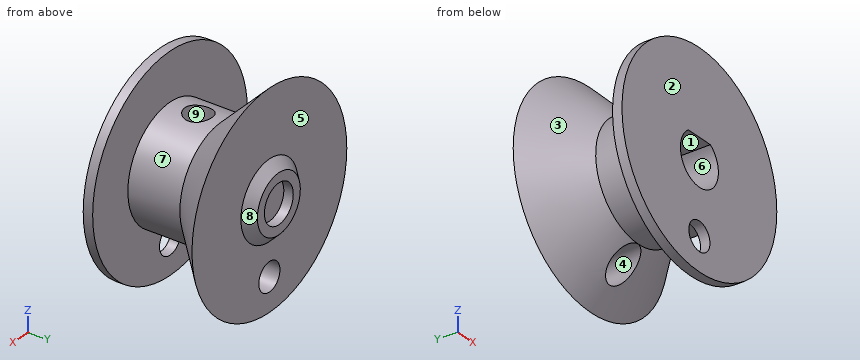
```python
from build123d import *

# Parameters (mm, degrees)
FLATSPOT_EXTRUDE_REACH     = 21.956
WIRE_HOLE_CUT_DEPTH        = 20.345542122
WIRE_HOLE_CUT_DEPTH_BACK   = 20.345542122
SKETCH5_R                  = 1.5
SKETCH6_R                  = 1.425
SET_SCREW_CUT_DEPTH        = 19.1400801
MAGNET_START               = -1
SKETCH8_R                  = 11
SKETCH8_R_2                = 3.05
MAGNET_HOLDER_TRIM_DEPTH   = 1
MAGNET_HOLDER_CHAMFER_SIZE = 1
AXLE_TOLERANCE_CUT_DEPTH   = 8


with BuildPart() as part:
    # Sketch1 → Spool Solid (revolve)
    with BuildSketch(Plane(origin=(0, 0, 0), x_dir=(0, 0, -1), z_dir=(1, 0, 0)), mode=Mode.PRIVATE) as spool_solid_sk:
        Polygon((-11, 6.25), (-11, 5.25), (-6, 0.25), (-6, -5.25), (-11, -5.25), (-11, -6.25), (-2.5, -6.25), (-2.5, 1.75), (0, 4.25), (0, 5.25), (-2.05, 5.25), (-2.05, 6.25), (-2.5, 6.25), align=None)
    revolve(spool_solid_sk.sketch.rotate(Axis((0, 0, 0), (0, 1, 0)), 180), axis=Axis((0, 0, 0), (0, 1, 0)))

    # Flatspot Extrude: up to this cone (the profile starts inside it)
    flatspot_extrude_end = Plane(origin=(0, -6.25, 0), z_dir=(0, -1, 0)).offset(-10.499999) * Cone(1e-06, 43.456, 43.455999, align=(Align.CENTER, Align.CENTER, Align.MIN), mode=Mode.PRIVATE)
    # Sketch2 → Flatspot Extrude (add, up to the surface)
    with BuildSketch(Plane.XZ.offset(6.25), mode=Mode.PRIVATE) as flatspot_extrude_sk1:
        with BuildLine():
            Line((1.5, 2), (-1.5, 2))
            ThreePointArc((-1.5, 2), (0, 2.5), (1.5, 2))
        make_face()
    flatspot_extrude_tool1 = extrude(flatspot_extrude_sk1.sketch, amount=-FLATSPOT_EXTRUDE_REACH, mode=Mode.PRIVATE) & flatspot_extrude_end
    add(flatspot_extrude_tool1.solids().sort_by_distance((0, -6.25, 2.20182))[0])

    # Sketch5 → Wire Hole cut (cut, two sides: drawn at the far end of the back side and taken through both)
    with BuildSketch(Plane(origin=(0, -5.25, 0), x_dir=(1, 0, 0), z_dir=(0, 1, 0)).offset(-WIRE_HOLE_CUT_DEPTH_BACK)):
        with Locations(Location((0, 7.5, 0), (0, 0, 270))):
            Circle(SKETCH5_R)
    extrude(amount=WIRE_HOLE_CUT_DEPTH + WIRE_HOLE_CUT_DEPTH_BACK, mode=Mode.SUBTRACT)

    # Sketch6 → Set Screw Cut (cut, through all)
    with BuildSketch(Plane(origin=(0, 0, 2), x_dir=(-1, 0, 0), z_dir=(0, 0, -1))):
        with Locations((0, -2.25)):
            Circle(SKETCH6_R)
    extrude(amount=-SET_SCREW_CUT_DEPTH, mode=Mode.SUBTRACT)

    # Sketch8 → Magnet Holder Trim (cut)
    with BuildSketch(Plane(origin=(0, 6.25, 0), x_dir=(1, 0, 0), z_dir=(0, 1, 0)).offset(MAGNET_START)):
        with Locations(Location((0, 0, 0), (0, 0, 90))):
            Circle(SKETCH8_R)
        with Locations(Location((0, 0, 0), (0, 0, 270))):
            Circle(SKETCH8_R_2, mode=Mode.SUBTRACT)
    extrude(amount=MAGNET_HOLDER_TRIM_DEPTH, mode=Mode.SUBTRACT)

    # Magnet Holder Chamfer
    magnet_holder_chamfer_edges = [part.edges().sort_by_distance(p)[0] for p in [
        (0, 5.25, -3.05),
    ]]
    chamfer(magnet_holder_chamfer_edges, length=MAGNET_HOLDER_CHAMFER_SIZE - 0.0001)  # a hair under: the kernel refuses the full size

    # Sketch9 → Axle Tolerance Cut (cut)
    with BuildSketch(Plane.XZ.offset(6.25)):
        with BuildLine():
            Line((1.565247584, 2.2), (-1.565247584, 2.2))
            ThreePointArc((-1.565247584, 2.2), (0, -2.7), (1.565247584, 2.2))
        make_face()
    extrude(amount=-AXLE_TOLERANCE_CUT_DEPTH, mode=Mode.SUBTRACT)


solid = part.part
```
CAD build for the part. Positions are in the model's coordinates, mm. Face numbers are marked on the shaded views. A direction names the side the tool comes from. Round coordinates to 2 decimals unless told otherwise and drop trailing zeros. Write each loop counter-clockwise with the first axis right and the second up, starting at its lowest first coordinate (ties: lowest second). Pieces come first, ordered by that corner, then holes. Notation, with made-up numbers: (82, -4) - (139, -4) arc R33 ccw to (139, 34) - close; hole circle Ø10 at (69.25, -1.75). An arc over 180 degrees is marked (long way). Return JSON: item names as keys, results as strings. Group by question number.
Item 1: Probe probe 1 along Y at (x, z) = (0, 10); probe 2 along Z at (x, y) = (0.25, 4.5); probe 3 along Y at (x, z) = (-7.25, -6.75). List the from-to ranges inside material, lowest first.
Item 2: Flat gauge pins, fed straight in: pin 1 Ø4 at (x, z) = (0, -7.5) entering from +Y; pin 2 Ø3.5 at (x, y) = (0, -2.25) entering from -Z; pin 3 Ø5 at (x, y) = (4.5, -5) entering from -Z. Where does each tip first touch, or does it go through?
Item 3: Band-saw the part on B-B on y = -2.25. List the corners of the cut face in (x, z) (3 decimals), plus the area to 3 significant figures.
Item 4: Mould opens along Y. For the marked faces 6, 7, 8 and 9 say: +Y half, -Y half, draft (parallel to the pull), parting line (faces both ways), or undercut.
Item 5: 3-axis set-ups, long thin cutter, end or side, ignore diameter. For the marked faces 1, 2, 3, 4 and 5: which of +Z, -Z, +X, -X, +Y, -Y reach the whole face in a straight line?
Item 6: Band-saw the part on A-A on z = -8. State how many separate pieces and enclosed holes the cut face has, plus the area to 3 significant figures.
Resolved:
{
 "1": {"probe 1": "y = -6.25 to -5.25, 4.25 to 5.25", "probe 2": "z = -10.25 to -8.98, -6.02 to 10.25", "probe 3": "y = -6.25 to -5.25, 4.16 to 5.25"},
 "2": {"pin 1": "stops at y = 5.25", "pin 2": "stops at z = -6", "pin 3": "stops at z = -10.81"},
 "3": {"outline": "(-1.565, 2.2) - (-1.425, 2.2) - (-1.425, 5.828) arc R6 ccw (long way) to (1.425, 5.828) - (1.425, 2.2) - (1.565, 2.2) arc R2.7 cw (long way) to start", "area": "80.6 mm²"},
 "4": {"face 6": "draft", "face 7": "undercut", "face 8": "+Y half", "face 9": "undercut"},
 "5": {"face 1": "-Y", "face 2": "+Z, -Z, +X, -X, -Y", "face 3": "none", "face 4": "+Y, -Y", "face 5": "+Y"},
 "6": {"separate pieces": "4", "enclosed holes": "0", "area": "33.1 mm²"}
}
